```python
from build123d import *

# Parameters (mm, degrees)
SKIZZE1_W                       = 100
SKIZZE1_H                       = 70
AUFSATZ_LINEAR_AUSTRAGEN1_DEPTH = 2
SKIZZE2_W                       = 80
SKIZZE2_H                       = 3
SKIZZE2_W_2                     = 3
SKIZZE2_H_2                     = 50
AUFSATZ_LINEAR_AUSTRAGEN2_DEPTH = 3
FASE1_SIZE                      = 1
SKIZZE3_R                       = 1.5
SCHNITT_LINEAR_AUSTRAGEN1_DEPTH = 123.102416029
SKIZZE4_W                       = 50
SKIZZE4_H                       = 26
SCHNITT_LINEAR_AUSTRAGEN2_DEPTH = 0.01
SKIZZE6_W                       = 50
SKIZZE6_H                       = 26
SCHNITT_LINEAR_AUSTRAGEN3_DEPTH = 1


with BuildPart() as part:
    # Skizze1 → Aufsatz-Linear austragen1 (new body)
    with BuildSketch(Plane.XY):
        with Locations((50, -35)):
            Rectangle(SKIZZE1_W, SKIZZE1_H)
    extrude(amount=AUFSATZ_LINEAR_AUSTRAGEN1_DEPTH)

    # Skizze2 → Aufsatz-Linear austragen2 (add)
    with BuildSketch(Plane.XY.offset(2)):
        with Locations((50, -3.5)):
            Rectangle(SKIZZE2_W, SKIZZE2_H)
        with Locations((50, -66.5)):
            Rectangle(SKIZZE2_W, SKIZZE2_H)
        with Locations((96.5, -35)):
            Rectangle(SKIZZE2_W_2, SKIZZE2_H_2)
        with Locations((3.5, -35)):
            Rectangle(SKIZZE2_W_2, SKIZZE2_H_2)
    extrude(amount=AUFSATZ_LINEAR_AUSTRAGEN2_DEPTH)

    # Fase1
    fase1_edges = [part.edges().sort_by_distance(p)[0] for p in [
        (50, -2, 5),
        (50, -68, 5),
        (98, -35, 5),
        (2, -35, 5),
    ]]
    chamfer(fase1_edges, length=FASE1_SIZE)

    # Skizze3 → Schnitt-Linear austragen1 (cut, through all)
    with BuildSketch(Plane.XY.offset(2)):
        with Locations((4, -4)):
            Circle(SKIZZE3_R)
        with Locations((96, -4)):
            Circle(SKIZZE3_R)
        with Locations((96, -66)):
            Circle(SKIZZE3_R)
        with Locations((4, -66)):
            Circle(SKIZZE3_R)
    extrude(amount=-SCHNITT_LINEAR_AUSTRAGEN1_DEPTH, mode=Mode.SUBTRACT)

    # Skizze4 → Schnitt-Linear austragen2 (cut)
    with BuildSketch(Plane(origin=(0, 0, 0), x_dir=(-1, 0, 0), z_dir=(0, 0, -1))):
        with Locations((-31, -45)):
            Rectangle(SKIZZE4_W, SKIZZE4_H)
    extrude(amount=-SCHNITT_LINEAR_AUSTRAGEN2_DEPTH, mode=Mode.SUBTRACT)

    # Skizze6 → Schnitt-Linear austragen3 (cut)
    with BuildSketch(Plane.XY.offset(2)):
        with Locations((31, -45)):
            Rectangle(SKIZZE6_W, SKIZZE6_H)
    extrude(amount=-SCHNITT_LINEAR_AUSTRAGEN3_DEPTH, mode=Mode.SUBTRACT)


solid = part.part
```
Geometry check sheet. Reference: the model listing, model coordinates, mm. A direction names the side the tool comes from. Round coordinates to 2 decimals unless told otherwise and drop trailing zeros. Loops run counter-clockwise (first coordinate to the right, second up) from the corner with the lowest first, then second, coordinate; pieces in that order, holes last. Notation, with made-up numbers: (53.5, 35.5) - (102.5, 35.5) arc R28 cw to (102.5, 65.5) - close; hole circle Ø3 at (27.5, 5.25). An arc over 180 degrees is marked (long way). Write item = value, one per line. Start each with the question number.
1. Depth check by flat-ended pin: pin 1 (2 mm diameter, centred on x = 61.5, z = 4, fed in from +Y); pin 2 (0.9 mm diameter, centred on y = -66.5, z = 3, fed in from -X); pin 3 (5 mm diameter, centred on x = 32, y = -9, fed in from +Z). Enter the tip coordinate at first touch or a pass-through.
2. Mould release check, pull along X, two halves, no side actions. Record for faces 6 (the face through (49, -2, 3)), 7 (the face through (90, -67, 3)), 8 (the face through (10, -4, 3)), 9 (the face through (97.43, -3.55, 1.01)): released by +X, released by -X, zero draft, split by the parting line, or undercut.
3. Set-up check for faces 1 (the face through (60, -35, 0)), 2 (the face through (49, -65, 3)), 3 (the face through (96, -10, 3)), 4 (the face through (49, 0, 1)), 5 (the face through (95, -35, 3)): record each of +Z, -Z, +X, -X, +Y, -Y from which the full face is reachable in a straight line by a thin tool's end or side.
4. Section check A-A on x = 96. Enter the section's corners in (y, z), then the cut area to 3 significant figures.
5. Section check B-B on y = -66. Enter the section's corners in (x, z).
6. Thickness scan on line 1 (X direction, y = -66, z = 1.45); line 2 (Y direction, x = 4, z = 1.15); line 3 (Y direction, x = 67.5, z = 2.6). Record the ranges inside material, lowest first.
7. Section check D-D on y = -19.5. Enter the section's corners in (x, z), then the cut area to 3 significant figures.
8. Section check C-C on x = 75.5. Enter the section's corners in (y, z).
Working result:
q1.pin_1 = -2
q1.pin_2 = 10
q1.pin_3 = 2
q2.face_6 = zero draft
q2.face_7 = released by +X
q2.face_8 = released by -X
q2.face_9 = undercut
q3.face_1 = -Z, +X, -X, +Y, -Y
q3.face_2 = +Z, +X, -X
q3.face_3 = +Z, +X, -X, +Y
q3.face_4 = +Z, -Z, +X, -X, +Y
q3.face_5 = +Z, +Y, -Y
q4.outline = (-70, 0) - (-67.5, 0) - (-67.5, 2) - (-70, 2) - close; (-64.5, 0) - (-5.5, 0) - (-5.5, 2) - (-10, 2) - (-10, 5) - (-60, 5) - (-60, 2) - (-64.5, 2) - close; (-2.5, 0) - (0, 0) - (0, 2) - (-2.5, 2) - close
q4.area = 278 mm^2
q5.outline = (0, 0) - (2.5, 0) - (2.5, 2) - (0, 2) - close; (5.5, 0) - (94.5, 0) - (94.5, 2) - (90, 2) - (90, 5) - (10, 5) - (10, 2) - (5.5, 2) - close; (97.5, 0) - (100, 0) - (100, 2) - (97.5, 2) - close
q6.line_1 = 0 to 2.5, 5.5 to 94.5, 97.5 to 100
q6.line_2 = -70 to -67.5, -64.5 to -5.5, -2.5 to 0
q6.line_3 = -68 to -65, -5 to -2
q7.outline = (0, 0) - (100, 0) - (100, 2) - (98, 2) - (98, 4) - (97, 5) - (95, 5) - (95, 2) - (5, 2) - (5, 5) - (3, 5) - (2, 4) - (2, 2) - (0, 2) - close
q7.area = 217 mm^2
q8.outline = (-70, 0) - (0, 0) - (0, 2) - (-2, 2) - (-2, 4) - (-3, 5) - (-5, 5) - (-5, 2) - (-65, 2) - (-65, 5) - (-67, 5) - (-68, 4) - (-68, 2) - (-70, 2) - close
